Model file for the job. Use its own axes, mm. Face numbers are marked on the shaded views. Round coordinates to 2 decimals unless told otherwise and drop trailing zeros. Use one line per item in the form item = value.
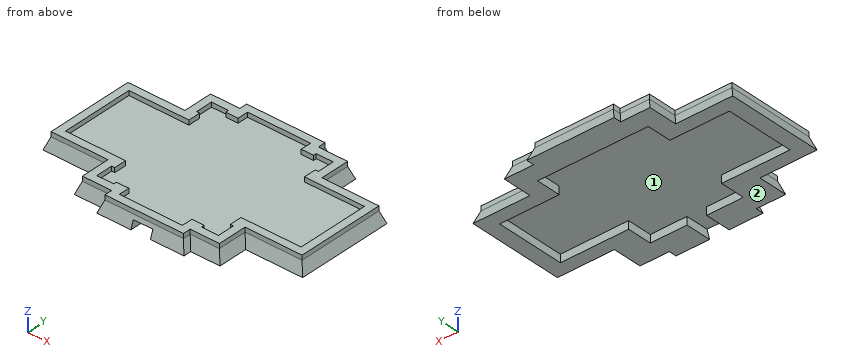
from build123d import *

# Parameters (mm, degrees)
F1_DEPTH = 3
F2_DEPTH = 7.62
F2_TAPER = -20
F4_DEPTH = 5.08


with BuildPart() as f1:
    # F0 (on Top) → F1 (new body)
    with BuildSketch(Plane.XY):
        Polygon((51.7914976329, 55.718055591), (32.7914976329, 55.718055591), (32.7914976329, 60.718055591), (7.2914976329, 60.718055591), (-18.2085023671, 60.718055591), (-18.2085023671, 55.718055591), (-37.2085023671, 55.718055591), (-37.2085023671, 36.718055591), (-74.2085023671, 36.718055591), (-74.2085023671, 8.218055591), (-74.2085023671, -20.281944409), (-37.2085023671, -20.281944409), (-37.2085023671, -39.281944409), (-18.2085023671, -39.281944409), (-18.2085023671, -44.281944409), (7.2914976329, -44.281944409), (32.7914976329, -44.281944409), (32.7914976329, -39.281944409), (51.7914976329, -39.281944409), (51.7914976329, -20.281944409), (88.7914976329, -20.281944409), (88.7914976329, 8.218055591), (88.7914976329, 36.718055591), (51.7914976329, 36.718055591), align=None)
        Polygon((-69.2085023671, 8.218055591), (-69.2085023671, 31.718055591), (-30.2085023671, 31.718055591), (-30.2085023671, 39.718055591), (-32.2085023671, 39.718055591), (-32.2085023671, 50.718055591), (-21.2085023671, 50.718055591), (-21.2085023671, 48.718055591), (-13.2085023671, 48.718055591), (-13.2085023671, 55.718055591), (7.2914976329, 55.718055591), (27.7914976329, 55.718055591), (27.7914976329, 48.718055591), (35.7914976329, 48.718055591), (35.7914976329, 50.718055591), (46.7914976329, 50.718055591), (46.7914976329, 39.718055591), (44.7914976329, 39.718055591), (44.7914976329, 31.718055591), (83.7914976329, 31.718055591), (83.7914976329, 8.218055591), (83.7914976329, -15.281944409), (44.7914976329, -15.281944409), (44.7914976329, -23.281944409), (46.7914976329, -23.281944409), (46.7914976329, -34.281944409), (35.7914976329, -34.281944409), (35.7914976329, -32.281944409), (27.7914976329, -32.281944409), (27.7914976329, -39.281944409), (7.2914976329, -39.281944409), (-13.2085023671, -39.281944409), (-13.2085023671, -32.281944409), (-21.2085023671, -32.281944409), (-21.2085023671, -34.281944409), (-32.2085023671, -34.281944409), (-32.2085023671, -23.281944409), (-30.2085023671, -23.281944409), (-30.2085023671, -15.281944409), (-69.2085023671, -15.281944409), align=None, mode=Mode.SUBTRACT)
    extrude(amount=F1_DEPTH)

    # F0 (on Top) → F2 (join)
    with BuildSketch(Plane.XY):
        Polygon((51.7914976329, 55.718055591), (32.7914976329, 55.718055591), (32.7914976329, 60.718055591), (7.2914976329, 60.718055591), (-18.2085023671, 60.718055591), (-18.2085023671, 55.718055591), (-37.2085023671, 55.718055591), (-37.2085023671, 36.718055591), (-74.2085023671, 36.718055591), (-74.2085023671, 8.218055591), (-74.2085023671, -20.281944409), (-37.2085023671, -20.281944409), (-37.2085023671, -39.281944409), (-18.2085023671, -39.281944409), (-18.2085023671, -44.281944409), (7.2914976329, -44.281944409), (32.7914976329, -44.281944409), (32.7914976329, -39.281944409), (51.7914976329, -39.281944409), (51.7914976329, -20.281944409), (88.7914976329, -20.281944409), (88.7914976329, 8.218055591), (88.7914976329, 36.718055591), (51.7914976329, 36.718055591), align=None)
        Polygon((-69.2085023671, 8.218055591), (-69.2085023671, 31.718055591), (-30.2085023671, 31.718055591), (-30.2085023671, 39.718055591), (-32.2085023671, 39.718055591), (-32.2085023671, 50.718055591), (-21.2085023671, 50.718055591), (-21.2085023671, 48.718055591), (-13.2085023671, 48.718055591), (-13.2085023671, 55.718055591), (7.2914976329, 55.718055591), (27.7914976329, 55.718055591), (27.7914976329, 48.718055591), (35.7914976329, 48.718055591), (35.7914976329, 50.718055591), (46.7914976329, 50.718055591), (46.7914976329, 39.718055591), (44.7914976329, 39.718055591), (44.7914976329, 31.718055591), (83.7914976329, 31.718055591), (83.7914976329, 8.218055591), (83.7914976329, -15.281944409), (44.7914976329, -15.281944409), (44.7914976329, -23.281944409), (46.7914976329, -23.281944409), (46.7914976329, -34.281944409), (35.7914976329, -34.281944409), (35.7914976329, -32.281944409), (27.7914976329, -32.281944409), (27.7914976329, -39.281944409), (7.2914976329, -39.281944409), (-13.2085023671, -39.281944409), (-13.2085023671, -32.281944409), (-21.2085023671, -32.281944409), (-21.2085023671, -34.281944409), (-32.2085023671, -34.281944409), (-32.2085023671, -23.281944409), (-30.2085023671, -23.281944409), (-30.2085023671, -15.281944409), (-69.2085023671, -15.281944409), align=None, mode=Mode.SUBTRACT)
        Polygon((-30.2085023671, 31.718055591), (-69.2085023671, 31.718055591), (-69.2085023671, 8.218055591), (-69.2085023671, -15.281944409), (-30.2085023671, -15.281944409), (-30.2085023671, -23.281944409), (-32.2085023671, -23.281944409), (-32.2085023671, -34.281944409), (-21.2085023671, -34.281944409), (-21.2085023671, -32.281944409), (-13.2085023671, -32.281944409), (-13.2085023671, -39.281944409), (7.2914976329, -39.281944409), (27.7914976329, -39.281944409), (27.7914976329, -32.281944409), (35.7914976329, -32.281944409), (35.7914976329, -34.281944409), (46.7914976329, -34.281944409), (46.7914976329, -23.281944409), (44.7914976329, -23.281944409), (44.7914976329, -15.281944409), (83.7914976329, -15.281944409), (83.7914976329, 8.218055591), (83.7914976329, 31.718055591), (44.7914976329, 31.718055591), (44.7914976329, 39.718055591), (46.7914976329, 39.718055591), (46.7914976329, 50.718055591), (35.7914976329, 50.718055591), (35.7914976329, 48.718055591), (27.7914976329, 48.718055591), (27.7914976329, 55.718055591), (7.2914976329, 55.718055591), (-13.2085023671, 55.718055591), (-13.2085023671, 48.718055591), (-21.2085023671, 48.718055591), (-21.2085023671, 50.718055591), (-32.2085023671, 50.718055591), (-32.2085023671, 39.718055591), (-30.2085023671, 39.718055591), align=None)
    extrude(amount=-F2_DEPTH, taper=F2_TAPER)

    # F3 (on face) → F4 (cut)
    with BuildSketch(Plane(origin=(0, 0, -7.62), x_dir=(1, 0, 0), z_dir=(0, 0, -1))):
        Polygon((-28.4716319293, 14.2964404076), (-67.0940428972, 14.2964404076), (-67.0940428972, -30.6183788925), (-28.4716319293, -30.6183788925), (-28.4716319293, -46.6748848557), (43.3486886322, -46.6748848557), (43.3486886322, -30.6183788925), (81.9710996002, -30.6183788925), (81.9710996002, 14.2964404076), (43.3486886322, 14.2964404076), (37.6397153199, 14.2964404076), (37.6397153199, 30.3529463708), (13.7885283515, 30.3529463708), (13.7885283515, 47.0553975941), (1.0885283515, 47.0553975941), (1.0885283515, 30.3529463708), (-22.7626586169, 30.3529463708), (-22.7626586169, 14.2964404076), align=None)
    extrude(amount=-F4_DEPTH, mode=Mode.SUBTRACT)


solid = f1.part
(1) Pin check, flat tips, straight feed: pin 1 (3.5 mm diameter, centred on x = -50.5, z = 2, fed in from -Y); pin 2 (4 mm diameter, centred on x = -3, y = -7, fed in from +Z); pin 3 (3 mm diameter, centred on x = 37.5, y = 37, fed in from -Z). Stop position of each tip, or through.
Report:
pin_1 = -20.28
pin_2 = 0
pin_3 = -2.54
(2) Probe probe 1 along Y at (x, z) = (-24.5, 1.75); probe 2 along X at (y, z) = (22, 2.25); probe 3 along Y at (x, z) = (-59, 0.5). List the from-to ranges inside material, lowest first. Write a range as [from, to].
Report:
probe_1 = [-39.28, -34.28], [50.72, 55.72]
probe_2 = [-74.21, -69.21], [83.79, 88.79]
probe_3 = [-20.28, -15.28], [31.72, 36.72]
(3) Pull direction Y, two halves, no side cores. Call the marked faces 1 and 2: released by +Y, released by -Y, zero draft, split by the parting line, or undercut.
Report:
face_1 = undercut
face_2 = zero draft
